```python
from build123d import *

# Parameters (mm, degrees)
F1_DEPTH = 6
F2_R     = 4
F3_DEPTH = 6
F4_R     = 0.4


with BuildPart() as f1:
    # F0 (on Front) → F1 (new body)
    with BuildSketch(Plane.XZ):
        Polygon((3.3950570152, -6.6937972181), (7.4945269462, -0.4066929865), (4.099469931, 6.2871042315), (-3.3950570152, 6.6937972181), (-7.4945269462, 0.4066929865), (-4.099469931, -6.2871042315), align=None)
    extrude(amount=F1_DEPTH)

    # F2 (on face) → F3 (intersect)
    with BuildSketch(Plane.XZ.offset(6)):
        Polygon((-7.4945269462, 0.4066929865), (-4.099469931, -6.2871042315), (3.3950570152, -6.6937972181), (7.4945269462, -0.4066929865), (4.099469931, 6.2871042315), (-3.3950570152, 6.6937972181), align=None)
        Circle(F2_R, mode=Mode.SUBTRACT)
    extrude(amount=-F3_DEPTH, mode=Mode.INTERSECT)

    # F4
    f4_edges = [f1.edges().sort_by_distance(p)[0] for p in [
        (-7.494527, -3, 0.406693),
        (-4.09947, -3, -6.287104),
        (-5.796998, 0, -2.940206),
        (-5.796998, -6, -2.940206),
        (3.395057, -3, -6.693797),
        (-0.352206, 0, -6.490451),
        (-0.352206, -6, -6.490451),
        (-3.395057, -3, 6.693797),
        (-5.444792, 0, 3.550245),
        (-5.444792, -6, 3.550245),
        (4.09947, -3, 6.287104),
        (0.352206, 0, 6.490451),
        (0.352206, -6, 6.490451),
        (7.494527, -3, -0.406693),
        (5.796998, 0, 2.940206),
        (5.796998, -6, 2.940206),
        (5.444792, 0, -3.550245),
        (5.444792, -6, -3.550245),
        (-4, -6, 0),
        (-4, 0, 0),
    ]]
    fillet(f4_edges, radius=F4_R)


solid = f1.part
```
Can you work these out from the model? Positions are in its coordinate system, mm. Coordinates: 2 decimals unless noted, no trailing zeros. Loops run counter-clockwise (first coordinate to the right, second up) from the corner with the lowest first, then second, coordinate; pieces in that order, holes last.
1) Thinking about a two-plate mould opening in Z: for faces 1 (the cylindrical face through (-0.867, -3.036, -3.905)), 2 (the cylindrical face through (-5.376, -5.88, 3.447)), 3 (the flat face through (-0.401, -2.964, -6.488)), which applies, pulls with the +Z half, pulls with the -Z half, needs draft (parallel to the pull), parting line crosses it, or undercut?
2) For pin 1 (1 mm diameter, centred on x = -2.5, y = -4, fed in from -Z); pin 2 (2 mm diameter, centred on y = -2, z = -2, fed in from -X); pin 3 (1 mm diameter, centred on y = -5, z = 4.5, fed in from +X), each with a flat end and sliding along its axis, tell me the tip position at first contact or that it passes through.
3) Imagine slicing it at A-A on y = -3.75. List the corners of the cut face in (x, z) for me.
4) I need wall thicknesses on probe 1 along Z at (x, y) = (0, -1.7); probe 2 along Y at (x, z) = (-3, -6); probe 3 along Z at (x, y) = (-3, -1). Which ranges of each line are inside material? Lowest first, please.
Completed:
1. face 1: undercut
1. face 2: pulls with the +Z half
1. face 3: pulls with the -Z half
2. pin 1: stops at z = -6.4
2. pin 2: stops at x = -6.78
2. pin 3: stops at x = 5.26
3. outline: (-7.39, 0.2) - (-4.2, -6.08) arc R0.4 ccw to (-3.87, -6.3) - (3.16, -6.68) arc R0.4 ccw to (3.52, -6.5) - (7.37, -0.6) arc R0.4 ccw to (7.39, -0.2) - (4.2, 6.08) arc R0.4 ccw to (3.87, 6.3) - (-3.16, 6.68) arc R0.4 ccw to (-3.52, 6.5) - (-7.37, 0.6) arc R0.4 ccw to start; hole circle Ø8 at (0, 0)
4. probe 1: z = -6.51 to -4, 4 to 6.51
4. probe 2: y = -6 to 0
4. probe 3: z = -6.35 to -2.65, 2.65 to 6.67
